Geometry: final body of the model. Coordinates: model frame, mm. A direction names the side the tool comes from. Coordinates: 2 decimals unless noted, no trailing zeros. Loops run counter-clockwise (first coordinate to the right, second up) from the corner with the lowest first, then second, coordinate; pieces in that order, holes last. Notation, with made-up numbers: M 37,88 L 53,88 A21 cw 53,116 Z; hole C 12.25,-36.75 d2. An arc over 180 degrees is marked long. Write each question's results on one line, items separated by ' | '. Start each with the question number.
Autodesk Inventor part; units mm, degrees
ref_plane "YZ Plane" through (0, 0, 0) normal (1, 0, 0) x (0, 1, 0)
ref_plane "XZ Plane" through (0, 0, 0) normal (0, 1, 0) x (-1, 0, 0)
ref_plane "XY Plane" through (0, 0, 0) normal (0, 0, 1) x (1, 0, 0)
sketch "Sketch1" plane through (0, 0, 0) normal (0, 0, 1) x (1, 0, 0)
  line L0 (0, 0) -> (160, 0)
  line L1 (160, 0) -> (160, -137.5)
  line L2 (160, -137.5) -> (0, -137.5)
  line L3 (0, -137.5) -> (0, 0)
  dimension "d0" = 160
  dimension "d1" = 137.5
extrude "Extrusion1" add sketch "Sketch1" along normal blind 10
sketch "Sketch2" plane through (0, 0, 10) normal (0, 0, 1) x (1, 0, 0)
  circle A0 centre (35, -12.5) radius 2.5
  circle A1 centre (35, -37.5) radius 2.5
  line L0 (160, 0) -> (0, 0)
  line L1 (0, 0) -> (0, -137.5)
  circle A2 centre (125, -12.5) radius 2.5
  circle A3 centre (125, -37.5) radius 2.5
  line L2 (160, -137.5) -> (160, 0)
  dimension "d4" = 5
  dimension "d5" = 5
  dimension "d6" = 12.5
  dimension "d7" = 25
  dimension "d8" = 35
  dimension "d9" = 5
  dimension "d10" = 5
  dimension "d11" = 35
extrude "Extrusion2" cut sketch "Sketch2" against normal through all
sketch "Sketch3" plane through (0, 0, 10) normal (0, 0, 1) x (1, 0, 0)
  circle A0 centre (125, -12.5) radius 2.5
  circle A1 centre (35, -12.5) radius 2.5
  circle A2 centre (35, -37.5) radius 2.5
  circle A3 centre (125, -37.5) radius 2.5
  line L0 (160, 0) -> (0, 0)
  line L1 (0, 0) -> (0, -137.5)
  line L2 (0, -137.5) -> (160, -137.5)
  line L3 (160, -137.5) -> (160, 0)
  line L4 (5, -132.5) -> (5, -5)
  line L5 (5, -5) -> (155, -5)
  line L6 (155, -5) -> (155, -132.5)
  line L7 (155, -132.5) -> (5, -132.5)
  dimension "d14" = 5
extrude "Extrusion3" add sketch "Sketch3" along normal blind 10 contours L3 L2 L1 L0
sketch "Sketch4" plane through (0, 0, 10) normal (0, 0, 1) x (1, 0, 0)
  line L0 (155, -5) -> (5, -5)
  line L1 (70, -5) -> (90, -5)
  line L2 (90, -5) -> (90, -20)
  line L3 (90, -20) -> (70, -20)
  line L4 (70, -20) -> (70, -5)
  line L5 (0, 0) -> (0, -137.5)
  dimension "d17" = 20
  dimension "d18" = 15
  dimension "d19" = 70
extrude "Extrusion4" cut sketch "Sketch4" against normal through all
sketch "Sketch5" plane through (5, -132.5, 10) normal (0, 1, 0) x (1, 0, 0)
  circle A0 centre (30, -5) radius 2.5
  circle A1 centre (120, -5) radius 2.5
  line L0 (30, -5) -> (120, -5) construction
  line L1 (-5, -10) -> (155, -10)
  point P0 (-5, 10)
  point P1 (75, -10)
  point P2 (75, -5)
  dimension "d22" = 5
  dimension "d23" = 5
  dimension "d24" = 5
  dimension "d25" = 90
extrude "Extrusion5" cut sketch "Sketch5" against normal through all
sketch "Sketch6" plane through (5, -132.5, 10) normal (0, 1, 0) x (1, 0, 0)
  line L0 (-5, -10) -> (155, -10)
  line L1 (65, -10) -> (85, -10)
  line L2 (85, -10) -> (85, 0)
  line L3 (85, 0) -> (65, 0)
  line L4 (65, 0) -> (65, -10)
  point P0 (-5, 10)
  point P1 (75, -10)
  point P2 (75, -10)
  dimension "d28" = 20
  dimension "d29" = 10
extrude "Extrusion6" cut sketch "Sketch6" against normal through all
sketch "Sketch7" plane through (0, 0, 10) normal (0, 0, 1) x (1, 0, 0)
  line L0 (70, -137.5) -> (70, -132.5)
  line L1 (70, -132.5) -> (5, -132.5)
  line L2 (5, -132.5) -> (5, -5)
  line L3 (5, -5) -> (155, -5)
  line L4 (155, -5) -> (155, -132.5)
  line L5 (155, -132.5) -> (90, -132.5)
  line L6 (90, -132.5) -> (90, -137.5)
  line L7 (90, -137.5) -> (160, -137.5)
  line L8 (160, -137.5) -> (160, 0)
  line L9 (160, 0) -> (0, 0)
  line L10 (0, 0) -> (0, -137.5)
  line L11 (0, -137.5) -> (70, -137.5)
  line L12 (5, -132.5) -> (5, -5)
  line L13 (5, -55) -> (155, -55)
  line L14 (5, -60) -> (155, -60)
  line L15 (155, -132.5) -> (155, -5)
  line L16 (5, -55) -> (5, -60)
  line L17 (155, -55) -> (155, -60)
  line L18 (5, -77.5) -> (155, -77.5)
  line L19 (155, -77.5) -> (155, -82.5)
  line L20 (155, -82.5) -> (5, -82.5)
  line L21 (5, -82.5) -> (5, -77.5)
  dimension "d32" = 5
  dimension "d33" = 50
  dimension "d34" = 5
  dimension "d35" = 50
extrude "Extrusion7" add sketch "Sketch7" along normal blind 10 contours L2 L18 L4 L20 | L2 L13 L4 L14
sketch "Sketch8" plane through (0, 0, 10) normal (0, 0, 1) x (1, 0, 0)
  line L0 (90, -5) -> (70, -5)
  line L1 (0, -137.5) -> (70, -137.5)
  line L2 (70, -5) -> (65, -5)
  line L3 (65, -5) -> (65, -137.5)
  line L4 (65, -137.5) -> (70, -137.5)
  line L5 (70, -137.5) -> (70, -5)
  line L6 (155, -5) -> (90, -5)
  line L7 (155, -132.5) -> (90, -132.5)
  line L8 (90, -5) -> (95, -5)
  line L9 (95, -5) -> (95, -132.5)
  line L10 (95, -132.5) -> (90, -132.5)
  line L11 (90, -132.5) -> (90, -5)
  point P0 (0, 0)
  dimension "d38" = 5
  dimension "d39" = 5
extrude "Extrusion8" add sketch "Sketch8" along normal blind 10
sketch "Sketch9" plane through (0, 0, 10) normal (0, 0, 1) x (1, 0, 0)
  line L0 (90, -137.5) -> (70, -137.5)
  line L1 (70, -137.5) -> (70, -20)
  line L2 (70, -20) -> (90, -20)
  line L3 (90, -20) -> (90, -137.5)
  point P0 (0, 0)
extrude "Extrusion9" cut sketch "Sketch9" along normal through all
sketch "Sketch10" plane through (0, 0, 10) normal (0, 0, 1) x (1, 0, 0)
  line L0 (5, -55) -> (5, -5)
  line L1 (5, -30) -> (30, -5)
  line L2 (5, -5) -> (65, -5)
  line L3 (5, -30) -> (5, -5)
  line L4 (5, -5) -> (30, -5)
  line L5 (155, -5) -> (155, -55)
  line L6 (155, -30) -> (130, -5)
  line L7 (95, -5) -> (155, -5)
  line L8 (5, -82.5) -> (5, -132.5)
  line L9 (5, -132.5) -> (65, -132.5)
  line L10 (95, -82.5) -> (95, -132.5)
  line L11 (95, -132.5) -> (155, -132.5)
  line L12 (155, -132.5) -> (155, -82.5)
  line L13 (155, -82.5) -> (95, -82.5)
  line L14 (70, -137.5) -> (70, -5)
  line L15 (70, -5) -> (90, -5)
  line L16 (90, -5) -> (90, -137.5)
  line L17 (90, -137.5) -> (160, -137.5)
  line L18 (160, -137.5) -> (160, 0)
  line L19 (160, 0) -> (0, 0)
  line L20 (0, 0) -> (0, -137.5)
  line L21 (0, -137.5) -> (70, -137.5)
  line L22 (95, -5) -> (155, -5)
  line L23 (155, -5) -> (155, -55)
  line L24 (155, -55) -> (95, -55)
  line L25 (95, -55) -> (95, -5)
  line L26 (95, -60) -> (155, -60)
  line L27 (155, -60) -> (155, -77.5)
  line L28 (155, -77.5) -> (95, -77.5)
  line L29 (95, -77.5) -> (95, -60)
  line L30 (65, -132.5) -> (5, -132.5)
  line L31 (5, -132.5) -> (5, -82.5)
  line L32 (65, -60) -> (65, -77.5)
  line L33 (65, -77.5) -> (5, -77.5)
  line L34 (5, -77.5) -> (5, -60)
  line L35 (5, -60) -> (65, -60)
  line L36 (95, -132.5) -> (95, -82.5)
  line L37 (95, -82.5) -> (155, -82.5)
  line L38 (155, -82.5) -> (155, -132.5)
  line L39 (155, -132.5) -> (95, -132.5)
  line L40 (65, -5) -> (65, -55)
  line L41 (65, -55) -> (5, -55)
  line L42 (5, -55) -> (5, -5)
  line L43 (5, -5) -> (65, -5)
  line L44 (130, -5) -> (155, -5)
  line L45 (155, -5) -> (155, -30)
  line L46 (5, -107.5) -> (30, -132.5)
  line L47 (5, -107.5) -> (5, -132.5)
  line L48 (5, -132.5) -> (30, -132.5)
  line L49 (155, -107.5) -> (130, -132.5)
  line L50 (130, -132.5) -> (155, -132.5)
  line L51 (155, -132.5) -> (155, -107.5)
  dimension "d44" = 30
  dimension "d45" = 30
  dimension "d47" = 30
  dimension "d48" = 30
  dimension "d49" = 30
  dimension "d50" = 30
  dimension "d51" = 30
  dimension "d52" = 30
extrude "Extrusion10" add sketch "Sketch10" along normal blind 10 contours L0 L2 L1 | L5 L6 L7 | L46 L9 L8 | L49 L12 L11
sketch "Sketch11" plane through (0, 0, 20) normal (0, 0, 1) x (1, 0, 0)
  circle A0 centre (9.525, -9.525) radius 2.5
  line L0 (0, 0) -> (160, 0) construction
  line L1 (160, 0) -> (160, -137.5) construction
  line L2 (0, 0) -> (160, 0) construction
  line L3 (160, 0) -> (160, -137.5) construction
  line L4 (160, -137.5) -> (0, -137.5) construction
  line L5 (0, -137.5) -> (0, 0) construction
  line L6 (9.525, -9.525) -> (150.475, -9.525) construction
  line L7 (150.475, -9.525) -> (150.475, -127.975) construction
  line L8 (150.475, -127.975) -> (9.525, -127.975) construction
  line L9 (9.525, -127.975) -> (9.525, -9.525) construction
  circle A1 centre (150.475, -9.525) radius 2.5
  circle A2 centre (150.475, -127.975) radius 2.5
  circle A3 centre (9.525, -127.975) radius 2.5
  dimension "d55" = 5
  dimension "d56" = 9.525
  dimension "d57" = 5
  dimension "d58" = 5
  dimension "d59" = 5
extrude "Extrusion11" cut sketch "Sketch11" against normal through all
properties part number "NA002" material "ABS Plastic"
Item 1: Section D-D, the plane y = -57.5. Return loops of the section in (x, z), plus the area to 3 significant figures.
Item 2: Section B-B, the plane y = -37.5. Return loops of the section in (x, z).
Item 3: Ray query, L1, parallel to Y at x = 35, z = 5.75; L2, parallel to X at y = -69.5, z = 18.75; L3, parallel to Y at x = 58, z = 12. Return the intervals inside material, ascending. Write a range as [from, to].
Item 4: Contact query for flat-ended pins moving along their axis: P1, Ø2, axis at x = 33, y = -69, coming from the +Z side; P2, Ø3, axis at x = 126.5, z = 8.5, coming from the +Y side. Output: stop coordinate, or through.
Item 5: Section A-A, the plane x = 125. Return loops of the section in (y, z).
Item 6: Pull-direction query (X, two-part tool) for faces 1 (the cylindrical face through (9.2, -125.496, 10.14)), 2 (the flat face through (160, -70, 10)), 3 (the flat face through (81, 0, 10)); classes: released by +X, released by -X, zero draft, split by the parting line, or undercut.
Item 7: Set-up query: faces 4 (the cylindrical face through (37.31, -13.46, 5.07)), 5 (the flat face through (125, -55, 15)), 6 (the cylindrical face through (127.385, -134.965, 14.249)). Return all of +Z, -Z, +X, -X, +Y, -Y with unobstructed straight access to the full face (end or side cutting, diameter ignored); none if empty.
Item 8: Section C-C, the plane x = 15. Return loops of the section in (y, z).
Solutions:
1) outline: M 0,0 L 160,0 L 160,20 L 90,20 L 90,10 L 70,10 L 70,20 L 0,20 Z | area: 3,000 mm²
2) outline: M 0,0 L 32.5,0 L 32.5,10 L 5,10 L 5,20 L 0,20 Z; M 37.5,0 L 122.5,0 L 122.5,10 L 95,10 L 95,20 L 90,20 L 90,10 L 70,10 L 70,20 L 65,20 L 65,10 L 37.5,10 Z; M 127.5,0 L 160,0 L 160,20 L 155,20 L 155,10 L 127.5,10 Z
3) L1: y = [-137.5, -40], [-35, -15], [-10, 0] | L2: x = [0, 5], [65, 70], [90, 95], [155, 160] | L3: y = [-137.5, -132.5], [-82.5, -77.5], [-60, -55], [-5, 0]
4) P1: stops at z = 10 | P2: stops at y = 0
5) outline: M -137.5,0 L -40,0 L -40,10 L -55,10 L -55,20 L -60,20 L -60,10 L -77.5,10 L -77.5,20 L -82.5,20 L -82.5,10 L -132.5,10 L -132.5,12.5 L -137.5,12.5 Z; M -137.5,17.5 L -132.5,17.5 L -132.5,20 L -137.5,20 Z; M -35,0 L -15,0 L -15,10 L -35,10 Z; M -10,0 L 0,0 L 0,20 L -5,20 L -5,10 L -10,10 Z
6) face 1: undercut | face 2: released by +X | face 3: zero draft
7) face 4: +Z, -Z | face 5: +Z | face 6: -Y
8) outline: M -137.5,0 L 0,0 L 0,20 L -20,20 L -20,10 L -55,10 L -55,20 L -60,20 L -60,10 L -77.5,10 L -77.5,20 L -82.5,20 L -82.5,10 L -117.5,10 L -117.5,20 L -137.5,20 Z
